```python
from build123d import *

# Parameters (mm, degrees)
BOSS_EXTRUDE1_DEPTH       = 17
SKETCH2_R                 = 2
BOSS_EXTRUDE2_DEPTH       = 6
F_3_0MM_DOWEL_HOLE1_D     = 3
F_3_0MM_DOWEL_HOLE1_DEPTH = 6
F_3_0MM_DOWEL_HOLE1_TIP   = 0.901290929


with BuildPart() as part:
    # Sketch1 → Boss-Extrude1 (new body)
    with BuildSketch(Plane.XY):
        Polygon((1.732050808, 3), (-1.732050808, 3), (-3.464101615, 0), (-1.732050808, -3), (1.732050808, -3), (3.464101615, 0), align=None)
    extrude(amount=BOSS_EXTRUDE1_DEPTH)

    # Sketch2 → Boss-Extrude2 (add)
    with BuildSketch(Plane.XY.offset(17)):
        Circle(SKETCH2_R)
    extrude(amount=BOSS_EXTRUDE2_DEPTH)

    # Ø3.0mm Dowel Hole1
    with Locations(Plane(origin=(0, 0, 0), x_dir=(-1, 0, 0), z_dir=(0, 0, -1))):
        with Locations((0, 0)):
            Hole(F_3_0MM_DOWEL_HOLE1_D / 2, depth=F_3_0MM_DOWEL_HOLE1_DEPTH)
            with Locations((0, 0, -(F_3_0MM_DOWEL_HOLE1_DEPTH + F_3_0MM_DOWEL_HOLE1_TIP / 2))):  # 118° drill point
                Cone(0, F_3_0MM_DOWEL_HOLE1_D / 2, F_3_0MM_DOWEL_HOLE1_TIP, mode=Mode.SUBTRACT)


solid = part.part
```
Can you work these out from the model? Positions are in its coordinate system, mm. A direction names the side the tool comes from. Coordinates: 2 decimals unless noted, no trailing zeros. Loops run counter-clockwise (first coordinate to the right, second up) from the corner with the lowest first, then second, coordinate; pieces in that order, holes last.
1) Imagine slicing it at A-A on z = 10.25. List the corners of the cut face in (x, y) for me.
2) Imagine slicing it at C-C on x = 2.25. List the corners of the cut face in (y, z) for me.
3) Thinking about a two-plate mould opening in X: for faces 4 (the flat face through (-2.6, 1.5, 8.4)), 5 (the conical face through (0.056, -0.254, 6.745)), 6 (the flat face through (0, -3, 8)), which applies, pulls with the +X half, pulls with the -X half, needs draft (parallel to the pull), parting line crosses it, or undercut?
4) For pin 1 (2 mm diameter, centred on x = -0.5, z = 18.5, fed in from +Y); pin 2 (2.5 mm diameter, centred on x = 0, y = 0, fed in from -Z), each with a flat end and sliding along its axis, tell me the tip position at first contact or that it passes through.
5) Which directions (+Z, -Z, +X, -X, +Y, -Y) give clear straight access to the entire face, cutting with the end or side of a thin tool? Please do faces 1 (the cylindrical face through (-1.5, 0.07, 3.04)), 2 (the flat face through (2.6, 1.5, 8.4)), 3 (the cylindrical face through (0, -2, 20)).
6) Imagine slicing it at B-B on y = 1.75. List the corners of the cut face in (x, z) for me, plus the area to 3 significant figures.
7) Imagine slicing it at D-D on z = 21. List the corners of the cut face in (x, y) for me, plus the area to 3 significant figures.
8) I need wall thicknesses on probe 1 along Y at (x, z) = (0, 1.35); probe 2 along Y at (x, z) = (-0.5, 4); probe 3 along Z at (x, y) = (-2.75, 1). Which ranges of each line are inside material? Lowest first, please.
Completed:
1. outline: (-3.46, 0) - (-1.73, -3) - (1.73, -3) - (3.46, 0) - (1.73, 3) - (-1.73, 3) - close
2. outline: (-2.1, 0) - (2.1, 0) - (2.1, 17) - (-2.1, 17) - close
3. face 4: pulls with the -X half
3. face 5: undercut
3. face 6: needs draft
4. pin 1: stops at y = 2
4. pin 2: stops at z = 6.15
5. face 1: -Z
5. face 2: +Z, -Z, +X, +Y
5. face 3: +Z
6. outline: (-2.45, 0) - (2.45, 0) - (2.45, 17) - (0.97, 17) - (0.97, 23) - (-0.97, 23) - (-0.97, 17) - (-2.45, 17) - close
6. area: 95.0 mm2
7. outline: circle Ø4 at (0, 0)
7. area: 12.6 mm2
8. probe 1: y = -3 to -1.5, 1.5 to 3
8. probe 2: y = -3 to -1.41, 1.41 to 3
8. probe 3: z = 0 to 17
